Autodesk Inventor part; units mm, degrees
ref_plane "YZ Plane" through (0, 0, 0) normal (1, 0, 0) x (0, 1, 0)
ref_plane "XZ Plane" through (0, 0, 0) normal (0, 1, 0) x (-1, 0, 0)
ref_plane "XY Plane" through (0, 0, 0) normal (0, 0, 1) x (1, 0, 0)
sketch "Sketch1" plane through (0, 0, 0) normal (0, 1, 0) x (-1, 0, 0)
  point P0 (0, 0)
sketch "Sketch2" plane through (0, 0, 0) normal (0, 1, 0) x (-1, 0, 0)
  line L0 (0, 0) -> (-950, 0)
  line L1 (-950, 0) -> (-950, -700)
  line L2 (-950, -700) -> (0, -700)
  line L3 (0, -700) -> (0, 0)
  dimension "d0" = 700
  dimension "d2" = 950
extrude "Extrusion1" add sketch "Sketch2" along normal blind 200
sketch "Sketch4" plane through (0, 200, 0) normal (0, 1, 0) x (1, 0, 0)
  line L0 (0, 0) -> (950, 0)
  line L1 (0, 700) -> (0, 0)
  line L2 (0, 0) -> (950, 0)
  line L3 (950, 0) -> (950, 700)
  line L4 (950, 700) -> (0, 700)
  line L5 (0, 700) -> (0, 0)
  line L6 (100, 100) -> (850, 100)
  line L7 (850, 100) -> (850, 600)
  line L8 (850, 600) -> (100, 600)
  line L9 (100, 600) -> (100, 100)
  line L10 (175, 275) -> (775, 275)
  line L11 (775, 275) -> (775, 425)
  line L12 (775, 425) -> (175, 425)
  line L13 (175, 425) -> (175, 275)
  line L14 (223.5, 323.5) -> (726.5, 323.5)
  line L15 (726.5, 323.5) -> (726.5, 376.5)
  line L16 (726.5, 376.5) -> (223.5, 376.5)
  line L17 (223.5, 376.5) -> (223.5, 323.5)
  line L18 (225, 325) -> (725, 325)
  line L19 (725, 325) -> (725, 375)
  line L20 (725, 375) -> (225, 375)
  line L21 (225, 375) -> (225, 325)
  dimension "d20" = 1.5
  dimension "d22" = 1.5
  dimension "d23" = 1.5
  dimension "d24" = 1.5
  dimension "d25" = 750
  dimension "d26" = 600
  dimension "d27" = 500
  dimension "d28" = 150
  dimension "d29" = 50
  dimension "d30" = 50
  dimension "d31" = 100
  dimension "d32" = 100
  dimension "d33" = 75
  dimension "d34" = 175
  dimension "d35" = 500
  dimension "d36" = 50
extrude "Extrusion3" add sketch "Sketch4" along normal blind 800 contours L17 L16 L15 L14
extrude "Extrusion4" add sketch "Sketch4" along normal blind 790 contours L13 L12 L11 L10
extrude "Extrusion5" add sketch "Sketch4" along normal blind 785 contours L9 L8 L7 L6
extrude "Extrusion6" add sketch "Sketch4" along normal blind 800 contours L1 L4 L3 L0
extrude "Extrusion7" add sketch "Sketch4" along normal blind 799 contours L21 L20 L19 L18
properties part number "UMD_Gas_Burner"
The listing builds one solid part. Answer for the finished solid, in the listing's coordinates (mm). Give positions to 0.01 mm unless a question says otherwise; leave off trailing zeros. Write each question's results on one line, items separated by ' | '.
Q1. A flat-ended cylindrical pin translates along its axis: P1, Ø15, axis at x = 556.5, z = -338, coming from the +Y side. Find the tip coordinate at first contact, or state that the pin passes through.
Output values:
P1: y = 999
Q2. Consider L1, parallel to Y at x = 228, z = -369; L2, parallel to Y at x = 791, z = -239.5. Determine where each line is inside the solid, lowest interval first. Write a range as from..to.
Output values:
L1: 0..999 | L2: 0..985
Q3. For a pull along Z with two mould halves and no side action, classify faces 1 (the flat face through (472, 999, -350)), 2 (the flat face through (482, 493, -700)), 3 (the flat face through (0, 493, -355)), 4 (the flat face through (471, 990, -384)) as released by +Z, released by -Z, zero draft, split by the parting line, or undercut.
Output values:
face 1: undercut | face 2: released by -Z | face 3: zero draft | face 4: undercut
